For this review, take the finished solid that the model builds, in its own axes (mm). A direction names the side the tool comes from. Give positions to 0.01 mm unless a question says otherwise; leave off trailing zeros. Answer in a Markdown table with one row per item.
```python
from build123d import *

# Parameters (mm, degrees)
CROQUIS1_RX             = 24
CROQUIS1_RY             = 11.39361319
SALIENTE_EXTRUIR1_DEPTH = 5


with BuildPart() as part:
    # Croquis1 → Saliente-Extruir1 (new body)
    with BuildSketch(Plane.XY):
        with Locations((0, 0)):
            Ellipse(CROQUIS1_RX, CROQUIS1_RY)
        with BuildLine():
            Line((-7, 2), (-4.582575695, 2))
            ThreePointArc((-4.582575695, 2), (5, 0), (-4.582575695, -2))
            Line((-4.582575695, -2), (-7, -2))
            Line((-7, -2), (-7, 2))
        make_face(mode=Mode.SUBTRACT)
    extrude(amount=SALIENTE_EXTRUIR1_DEPTH)


solid = part.part
```
1. Wall thickness on line 1 (X direction, y = 0, z = 3.2); line 2 (Y direction, x = 0, z = 1.85); line 3 (X direction, y = 4, z = 0.65): over which ranges is each line inside the solid? List them lowest first. Write a range as [from, to].
Values:
| item | result |
|---|---|
| line 1 | x = [-24, -7], [5, 24] |
| line 2 | y = [-11.39, -5], [5, 11.39] |
| line 3 | x = [-22.47, -3], [3, 22.47] |
2. Mouldability with a two-part tool opening along Y and no side actions: class faces 3 (the face through (5, 0, 2)), 4 (the face through (-6, 2, 2)), 5 (the face through (5, -2, 0)) as released by +Y, released by -Y, zero draft, split by the parting line, or undercut.
Values:
| item | result |
|---|---|
| face 3 | undercut |
| face 4 | undercut |
| face 5 | zero draft |
3. For faces 1 (the face through (5, -2, 5)), 2 (the face through (-6, -2, 2)), list the 3-axis set-ups (+Z, -Z, +X, -X, +Y, -Y) from which the entire face can be reached by the end or side of a thin tool; tool diameter is ignored.
Values:
| item | result |
|---|---|
| face 1 | +Z, +X, -X, +Y, -Y |
| face 2 | +Z, -Z |
4. Clearance check with flat-ended pins moving along their axes: pin 1 (1.5 mm diameter, centred on x = -16.5, z = 2.5, fed in from +Y); pin 2 (2 mm diameter, centred on x = -6, z = 2, fed in from -Y); pin 3 (3 mm diameter, centred on x = -11, z = 2.5, fed in from +Y). State where each tip first meets the part, or that it passes through.
Values:
| item | result |
|---|---|
| pin 1 | stops at y = 8.6 |
| pin 2 | stops at y = -11.14 |
| pin 3 | stops at y = 10.46 |
